Check sheet for the modelled part. Datum: model origin and axes. Units: mm. Face numbers are marked on the shaded views. A direction names the side the tool comes from. Round coordinates to 2 decimals unless told otherwise and drop trailing zeros. Order: outer loops, then holes, each group sorted by start corner. A loop starts at its lowest first (then second) coordinate and runs counter-clockwise, first axis right, second up. Notation, with made-up numbers: (-21, 31.25) -> (26, 31.25) arc R35 cw to (26, 68.25) -> close; hole circle Ø1 at (70.25, 56.25). An arc over 180 degrees is marked (long way). Answer in a Markdown table with one row per item. Add a question column.
1. Depth check by flat-ended pin: P1, Ø6, axis at x = 76.52, z = -79.67, coming from the -Y side; P2, Ø3, axis at x = -29, y = -1.5, coming from the -Z side; P3, Ø2, axis at y = -9, z = -32, coming from the -X side; P4, Ø1, axis at x = 61, y = -7, coming from the -Z side. Enter the tip coordinate at first touch or a pass-through.
2. Access from +Z, -Z, +X, -X, +Y, -Y to the whole of each face (thin tool, end or side, straight path). Record for the marked faces 1 and 2.
3. Draft check along X on the marked faces 3, 4 and 5. Enter one of: +X half, -X half, draft (parallel to the pull), parting line (faces both ways), or undercut.
4. Material ranges on L1, parallel to Z at x = 69.5, y = -10.5; L2, parallel to X at y = -11.5, z = -2; L3, parallel to Z at x = -61.5, y = -1.25, recorded low to high. Write a range as from..to.
5. Sectioned sample at A-A, the plane z = -27.5. Record the boundary of the cut face in (x, y), then the cut area to 3 significant figures.
6. Sectioned sample at C-C, the plane y = -4.75. Count the separate pieces of the cut face and the enclosed holes in it, then the cut area to 3 significant figures.
7. Sectioned sample at B-B, the plane x = -9. Record the boundary of the cut face in (y, z), then the cut area to 3 significant figures.
```python
from build123d import *

# Parameters (mm, degrees)
F0_R     = 3.2639
F0_R_2   = 1.7018
F0_R_3   = 17.9959
F1_DEPTH = 12.7
F2_W     = 107.95
F2_H     = 19.1731796932
F3_DEPTH = 25.4
F4_F1_R  = 6.35
F4_F2_R  = 6.35
F5_R     = 6.35
F6_SIZE  = 0.508


# Not quite as in the source:
# - a feature names something its author has since deleted; it is built from what else it names


with BuildPart() as f1:
    # F0 (on Front) → F1 (new body)
    with BuildSketch(Plane.XZ):
        Polygon((-126.667948618, -98.8461842824), (95.582051382, -98.5286048876), (95.582051382, -60.4286048876), (95.582051382, -50.9036048876), (19.382051382, -50.9036048876), (19.382051382, -60.4286048876), (-18.717948618, -60.4286048876), (-18.717948618, 66.2538157176), (-126.667948618, 66.2538157176), align=None)
        with Locations((-66.3308787224, -79.5945032566)):
            Circle(F0_R, mode=Mode.SUBTRACT)
        with Locations((-37.7828981478, -79.6691544378)):
            Circle(F0_R, mode=Mode.SUBTRACT)
        with Locations((-66.3853614397, -41.4661356021)):
            Circle(F0_R, mode=Mode.SUBTRACT)
        with Locations((-37.7829381848, -41.4661356021)):
            Circle(F0_R, mode=Mode.SUBTRACT)
        with Locations((0.3171018521, -79.6691544378)):
            Circle(F0_R, mode=Mode.SUBTRACT)
        with Locations((38.4171018521, -79.6691544378)):
            Circle(F0_R, mode=Mode.SUBTRACT)
        with Locations((76.5171018521, -79.6691544378)):
            Circle(F0_R, mode=Mode.SUBTRACT)
        with Locations((-117.9733242227, -10.6661073038)):
            Circle(F0_R_2, mode=Mode.SUBTRACT)
        with Locations((-94.4033242227, -9.0925073038)):
            Circle(F0_R_2, mode=Mode.SUBTRACT)
        with Locations((-116.3997242227, 12.9038926962)):
            Circle(F0_R_2, mode=Mode.SUBTRACT)
        with Locations((-94.4033242227, 12.9038926962)):
            Circle(F0_R_3, mode=Mode.SUBTRACT)
        with Locations((-72.4069242227, 12.9038926962)):
            Circle(F0_R_2, mode=Mode.SUBTRACT)
        with Locations((-70.8333242227, -10.6661073038)):
            Circle(F0_R_2, mode=Mode.SUBTRACT)
        with Locations((-37.7829381848, -3.3661356021)):
            Circle(F0_R, mode=Mode.SUBTRACT)
        with Locations((-117.9733242227, 36.4738926962)):
            Circle(F0_R_2, mode=Mode.SUBTRACT)
        with Locations((-94.4033242227, 34.9002926962)):
            Circle(F0_R_2, mode=Mode.SUBTRACT)
        with Locations((-70.8333242227, 36.4738926962)):
            Circle(F0_R_2, mode=Mode.SUBTRACT)
    extrude(amount=F1_DEPTH)

    # F2 (on face) → F3 (cut)
    with BuildSketch(Plane.XZ.offset(12.7)):
        Polygon((-82.2600983048, -40.9187248283), (-126.667948618, -22.6552803069), (-126.667948618, -98.8461842824), (-82.2600983048, -98.7827286323), align=None)
        with Locations((-72.692948618, 56.6672258711)):
            Rectangle(F2_W, F2_H)
    extrude(amount=-F3_DEPTH, mode=Mode.SUBTRACT)

    # F4: fillet of radius 6.35 on 9 edges, made by hand

    # F4_f1
    f4_f1_edges = [f1.edges().sort_by_distance(p)[0] for p in [
        (-82.2600983048, -6.35, -40.9187248283),
        (-18.717948618, -6.35, -60.4286048876),
    ]]
    fillet(f4_f1_edges, radius=F4_F1_R)

    # F4_f2
    f4_f2_edges = [f1.edges().sort_by_distance(p)[0] for p in [
        (-126.667948618, -6.35, 47.0806360245),
        (-126.667948618, -6.35, -22.6552803069),
        (-18.717948618, -6.35, 47.0806360245),
        (-82.2600983048, -6.35, -98.7827286323),
        (95.582051382, -6.35, -98.5286048876),
        (95.582051382, -6.35, -50.9036048876),
        (19.382051382, -6.35, -50.9036048876),
    ]]
    fillet(f4_f2_edges, radius=F4_F2_R)

    # F5
    f5_edges = [f1.edges().sort_by_distance(p)[0] for p in [
        (19.382051, -6.35, -60.428605),
    ]]
    fillet(f5_edges, radius=F5_R)

    # F6
    f6_edges = [f1.edges().sort_by_distance(p)[0] for p in [
        (21.843486, -12.7, -52.233489),
        (17.323894, -12.7, -59.098721),
        (57.482051, -12.7, -50.903605),
        (0.53369, -12.7, -60.428605),
        (93.722179, -12.7, -52.763477),
        (-16.858077, -12.7, -58.568733),
        (95.582051, -12.7, -74.720638),
        (-18.717949, -12.7, -6.673984),
        (93.725386, -12.7, -96.674591),
        (-20.577821, -12.7, 45.220764),
        (6.67005, -12.7, -98.655654),
        (-72.692949, -12.7, 47.080636),
        (-80.397017, -12.7, -96.916983),
        (-124.808077, -12.7, 45.220764),
        (-82.260098, -12.7, -68.798442),
        (-126.667949, -12.7, 11.164933),
        (-83.334713, -12.7, -41.638718),
        (-125.593334, -12.7, -21.935287),
        (-104.464023, -12.7, -31.787003),
        (-69.594779, -12.7, -79.594503),
        (-41.046798, -12.7, -79.669154),
        (-69.649261, -12.7, -41.466136),
        (-41.046838, -12.7, -41.466136),
        (-2.946798, -12.7, -79.669154),
        (35.153202, -12.7, -79.669154),
        (73.253202, -12.7, -79.669154),
        (-119.675124, -12.7, -10.666107),
        (-96.105124, -12.7, -9.092507),
        (-72.535124, -12.7, -10.666107),
        (-41.046838, -12.7, -3.366136),
        (-118.101524, -12.7, 12.903893),
        (-112.399224, -12.7, 12.903893),
        (-74.108724, -12.7, 12.903893),
        (-119.675124, -12.7, 36.473893),
        (-96.105124, -12.7, 34.900293),
        (-72.535124, -12.7, 36.473893),
        (21.843486, 0, -52.233489),
        (17.323894, 0, -59.098721),
        (57.482051, 0, -50.903605),
        (0.53369, 0, -60.428605),
        (93.722179, 0, -52.763477),
        (-16.858077, 0, -58.568733),
        (95.582051, 0, -74.720638),
        (-18.717949, 0, -6.673984),
        (93.725386, 0, -96.674591),
        (-20.577821, 0, 45.220764),
        (6.67005, 0, -98.655654),
        (-72.692949, 0, 47.080636),
        (-80.397017, 0, -96.916983),
        (-124.808077, 0, 45.220764),
        (-82.260098, 0, -68.798442),
        (-126.667949, 0, 11.164933),
        (-83.334713, 0, -41.638718),
        (-125.593334, 0, -21.935287),
        (-104.464023, 0, -31.787003),
        (-69.594779, 0, -79.594503),
        (-41.046798, 0, -79.669154),
        (-69.649261, 0, -41.466136),
        (-41.046838, 0, -41.466136),
        (-2.946798, 0, -79.669154),
        (35.153202, 0, -79.669154),
        (73.253202, 0, -79.669154),
        (-119.675124, 0, -10.666107),
        (-96.105124, 0, -9.092507),
        (-72.535124, 0, -10.666107),
        (-41.046838, 0, -3.366136),
        (-118.101524, 0, 12.903893),
        (-112.399224, 0, 12.903893),
        (-74.108724, 0, 12.903893),
        (-119.675124, 0, 36.473893),
        (-96.105124, 0, 34.900293),
        (-72.535124, 0, 36.473893),
    ]]
    chamfer(f6_edges, length=F6_SIZE)


solid = f1.part
```
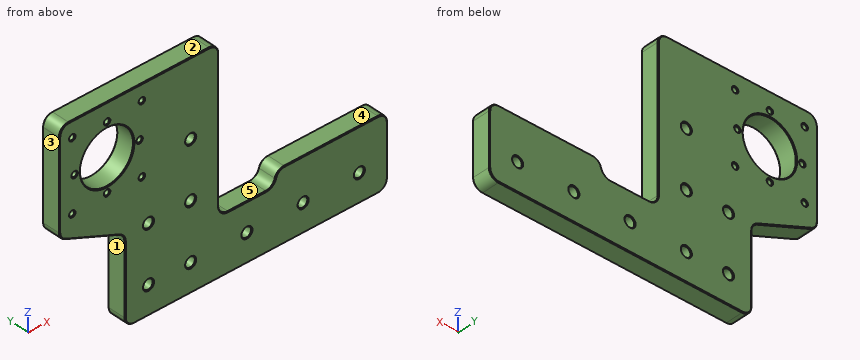
Answer key:
| question | item | result |
|---|---|---|
| 1 | P1 | passes through |
| 1 | P2 | stops at z = -98.71 |
| 1 | P3 | stops at x = -106.38 |
| 1 | P4 | stops at z = -98.58 |
| 2 | face 1 | -Z, -X, +Y, -Y |
| 2 | face 2 | +Z, +X, -X, +Y, -Y |
| 3 | face 3 | -X half |
| 3 | face 4 | draft |
| 3 | face 5 | undercut |
| 4 | L1 | z = -98.57..-50.9 |
| 4 | L2 | x = -126.67..-104.49, -84.32..-40.75, -34.82..-18.72 |
| 4 | L3 | z = -98.75..47.08 |
| 5 | outline | (-114.89, -12.19) -> (-113.55, -12.7) -> (-19.23, -12.7) -> (-18.72, -12.19) -> (-18.72, -0.51) -> (-19.23, 0) -> (-113.55, 0) -> (-114.89, -0.51) -> close |
| 5 | area | 1,220 mm² |
| 6 | separate pieces | 1 |
| 6 | enclosed holes | 17 |
| 6 | area | 16,500 mm² |
| 7 | outline | (-12.7, -98.17) -> (-12.19, -98.68) -> (-0.51, -98.68) -> (0, -98.17) -> (0, -60.94) -> (-0.51, -60.43) -> (-12.19, -60.43) -> (-12.7, -60.94) -> close |
| 7 | area | 485 mm² |
